Check sheet for the modelled part. Datum: model origin and axes. Units: mm. A direction names the side the tool comes from. Coordinates: 2 decimals unless noted, no trailing zeros. Order: outer loops, then holes, each group sorted by start corner. A loop starts at its lowest first (then second) coordinate and runs counter-clockwise, first axis right, second up. Notation, with made-up numbers: M -4.75,-9 L 16.25,-9 A14 ccw 16.25,8 Z; hole C 56,-18.5 d11. An arc over 180 degrees is marked long. Answer in a Markdown table with one row per item. Add a question column.
Autodesk Inventor part; units mm, degrees
ref_plane "YZ Plane" through (0, 0, 0) normal (1, 0, 0) x (0, 1, 0)
ref_plane "XZ Plane" through (0, 0, 0) normal (0, 1, 0) x (-1, 0, 0)
ref_plane "XY Plane" through (0, 0, 0) normal (0, 0, 1) x (1, 0, 0)
sketch "Sketch1" plane through (0, 0, 0) normal (0, 1, 0) x (-1, 0, 0)
  line L0 (-38.1, 0) -> (0, 0)
  line L1 (0, 0) -> (0, 38.1)
  line L2 (-34.925, 3.175) -> (-6.35, 3.175)
  line L3 (-3.175, 6.35) -> (-3.175, 34.925)
  line L4 (0, 38.1) -> (0, 38.1)
  line L5 (-38.1, 0) -> (-38.1, 0)
  arc A0 (0, 38.1) -> (-3.175, 34.925) centre (0, 34.925) ccw
  arc A1 (-34.925, 3.175) -> (-38.1, 0) centre (-34.925, 0) ccw
  arc A2 (-6.35, 3.175) -> (-3.175, 6.35) centre (-6.35, 6.35) ccw
  point P0 (0, 38.1)
  dimension "d0" = 38.1
  dimension "d1" = 38.1
  dimension "d2" = 3.175
  dimension "d3" = 3.175
extrude "Extrusion1" add sketch "Sketch1" along normal blind 50.8
sketch "Sketch2" plane through (38.1, 0, 0) normal (0, 0, -1) x (-1, 0, 0)
  line L0 (0, 0) -> (38.1, 0)
  line L1 (38.1, 0) -> (38.1, 50.8)
  line L2 (0, 50.8) -> (38.1, 50.8)
  line L3 (0, 0) -> (0, 50.8)
  point P0 (19.05, 38.1)
  point P1 (19.05, 12.7)
  dimension "d6" = 12.7
  dimension "d7" = 12.7
  dimension "d8" = 19.05
hole "Hole1" at (19.05, 38.1, 0) at (19.05, 12.7, 0) direction (0, 0, 1) diameter 5 end through all
sketch "Sketch3" plane through (0, 0, 0) normal (-1, 0, 0) x (0, 0, 1)
  line L0 (0, 0) -> (38.1, 0)
  line L1 (38.1, 0) -> (38.1, 50.8)
  line L2 (0, 50.8) -> (38.1, 50.8)
  line L3 (0, 0) -> (0, 50.8)
  point P0 (19.05, 38.1)
  point P1 (19.05, 12.7)
  dimension "d16" = 12.7
  dimension "d17" = 12.7
  dimension "d18" = 19.05
hole "Hole2" at (0, 38.1, 19.05) at (0, 12.7, 19.05) direction (1, 0, 0) diameter 5 end through all
properties part number "NASA-20-EBOX-EXT-CB-01"
1. Section check C-C on y = 12.7. Enter the section's corners in (x, z) (3 decimals), then the cut area to 3 significant figures.
2. Section check A-A on x = 19.05. Enter the section's corners in (y, z) (3 decimals).
3. Section check B-B on z = 19.05. Enter the section's corners in (x, y) (3 decimals), then the cut area to 3 significant figures.
4. Section check D-D on x = 32.5. Enter the section's corners in (y, z) (3 decimals).
5. Go/stop test with flat-tipped pins: pin 1 Ø14.5 at (y, z) = (38, 27.5) entering from +X (3 decimals); pin 2 Ø14.5 at (x, y) = (23, 17.5) entering from +Z (3 decimals). Record where each tip stops, or that it passes through.
6. Set-up check for faces 1 (the flat face through (0, 25, 19)), 2 (the flat face through (21, 25, 3.175)): record each of +Z, -Z, +X, -X, +Y, -Y from which the full face is reachable in a straight line by a thin tool's end or side.
7. Release check for a two-part mould opening along X. For faces 3 (the cylindrical face through (20.571, 36.116, 1.61)), 4 (the cylindrical face through (21.27, 13.85, 1.61)), 5 (the flat face through (3.175, 25, 20)), 6 (the flat face through (19, 25, 0)) record: released by +X, released by -X, zero draft, split by the parting line, or undercut.
8. Scan lines: line 1 (Y direction, x = 1.05, z = 19.05); line 2 (X direction, y = 43, z = 31) (3 decimals); line 3 (Z direction, x = 0.85, y = 12.7). Record each from-to range of solid material in increasing order.
Result sheet:
| question | item | result |
|---|---|---|
| 1 | outline | M 0,0 L 16.55,0 L 16.55,3.175 L 6.35,3.175 A3.175 cw 3.175,6.35 L 3.175,16.55 L 0,16.55 Z; M 0,21.55 L 3.175,21.55 L 3.175,34.925 A3.175 ccw 0,38.1 Z; M 21.55,0 L 38.1,0 A3.175 ccw 34.925,3.175 L 21.55,3.175 Z |
| 1 | area | 198 mm^2 |
| 2 | outline | M 0,0 L 10.2,0 L 10.2,3.175 L 0,3.175 Z; M 15.2,0 L 35.6,0 L 35.6,3.175 L 15.2,3.175 Z; M 40.6,0 L 50.8,0 L 50.8,3.175 L 40.6,3.175 Z |
| 3 | outline | M 0,0 L 3.175,0 L 3.175,10.2 L 0,10.2 Z; M 0,15.2 L 3.175,15.2 L 3.175,35.6 L 0,35.6 Z; M 0,40.6 L 3.175,40.6 L 3.175,50.8 L 0,50.8 Z |
| 3 | area | 130 mm^2 |
| 4 | outline | M 0,0 L 50.8,0 L 50.8,3.175 L 0,3.175 Z |
| 5 | pin 1 | x = 3.175 |
| 5 | pin 2 | z = 3.175 |
| 6 | face 1 | +Z, -Z, -X, +Y, -Y |
| 6 | face 2 | +Z, +X, +Y, -Y |
| 7 | face 3 | undercut |
| 7 | face 4 | undercut |
| 7 | face 5 | released by +X |
| 7 | face 6 | zero draft |
| 8 | line 1 | 0 to 10.2, 15.2 to 35.6, 40.6 to 50.8 |
| 8 | line 2 | 0 to 3.175 |
| 8 | line 3 | 0 to 16.55, 21.55 to 37.98 |
